```python
from build123d import *

# Parameters (mm, degrees)
BOSS_EXTRUDE1_DEPTH = 6.35
SKETCH2_R           = 1.5875
SKETCH2_W           = 80.264
SKETCH2_H           = 12.954
CUT_EXTRUDE1_DEPTH  = 224.053407282
SKETCH7_R           = 2.032
SKETCH7_R_2         = 1.651
SKETCH7_W           = 47.244
SKETCH7_H           = 139.192
CUT_EXTRUDE4_DEPTH  = 224.053407282
SKETCH8_R           = 1.651
CUT_EXTRUDE5_DEPTH  = 224.053407282
SKETCH9_R           = 1.778
CUT_EXTRUDE6_DEPTH  = 221.551312535


with BuildPart() as part:
    # Sketch1 → Boss-Extrude1 (new body)
    with BuildSketch(Plane(origin=(0, 0, 0), x_dir=(1, 0, 0), z_dir=(0, 1, 0))):
        with BuildLine():
            Line((-80, 112.5), (100, 112.5))
            Line((100, 112.5), (100, -112.5))
            Line((100, -112.5), (-80, -112.5))
            ThreePointArc((-80, -112.5), (-192.5, 0), (-80, 112.5))
        make_face()
    extrude(amount=-BOSS_EXTRUDE1_DEPTH)

    # Sketch2 → Cut-Extrude1 (cut, through all)
    with BuildSketch(Plane(origin=(0, 0, 0), x_dir=(1, 0, 0), z_dir=(0, 1, 0))):
        with Locations(Location((36.144045702, -66.3448, 0), (0, 0, 270))):
            Circle(SKETCH2_R)
        with Locations(Location((36.144045702, -59.9948, 0), (0, 0, 270))):
            Circle(SKETCH2_R)
        with Locations(Location((36.144045702, -53.6448, 0), (0, 0, 270))):
            Circle(SKETCH2_R)
        with Locations(Location((36.144045702, -47.2948, 0), (0, 0, 270))):
            Circle(SKETCH2_R)
        with Locations(Location((36.144045702, -40.9448, 0), (0, 0, 270))):
            Circle(SKETCH2_R)
        with Locations(Location((36.144045702, -34.5948, 0), (0, 0, 270))):
            Circle(SKETCH2_R)
        with Locations(Location((36.144045702, -28.2448, 0), (0, 0, 270))):
            Circle(SKETCH2_R)
        with Locations(Location((67.894045702, -66.3448, 0), (0, 0, 270))):
            Circle(SKETCH2_R)
        with Locations(Location((67.894045702, -59.9948, 0), (0, 0, 270))):
            Circle(SKETCH2_R)
        with Locations(Location((67.894045702, -53.6448, 0), (0, 0, 270))):
            Circle(SKETCH2_R)
        with Locations(Location((67.894045702, -47.2948, 0), (0, 0, 270))):
            Circle(SKETCH2_R)
        with Locations(Location((67.894045702, -40.9448, 0), (0, 0, 270))):
            Circle(SKETCH2_R)
        with Locations(Location((67.894045702, -34.5948, 0), (0, 0, 270))):
            Circle(SKETCH2_R)
        with Locations(Location((67.894045702, -28.2448, 0), (0, 0, 270))):
            Circle(SKETCH2_R)
        with Locations(Location((36.144045702, 66.3448, 0), (0, 0, 270))):
            Circle(SKETCH2_R)
        with Locations(Location((36.144045702, 59.9948, 0), (0, 0, 270))):
            Circle(SKETCH2_R)
        with Locations(Location((36.144045702, 53.6448, 0), (0, 0, 270))):
            Circle(SKETCH2_R)
        with Locations(Location((36.144045702, 47.2948, 0), (0, 0, 270))):
            Circle(SKETCH2_R)
        with Locations(Location((36.144045702, 40.9448, 0), (0, 0, 270))):
            Circle(SKETCH2_R)
        with Locations(Location((36.144045702, 34.5948, 0), (0, 0, 270))):
            Circle(SKETCH2_R)
        with Locations(Location((36.144045702, 28.2448, 0), (0, 0, 270))):
            Circle(SKETCH2_R)
        with Locations(Location((67.894045702, 66.3448, 0), (0, 0, 270))):
            Circle(SKETCH2_R)
        with Locations(Location((67.894045702, 59.9948, 0), (0, 0, 270))):
            Circle(SKETCH2_R)
        with Locations(Location((67.894045702, 53.6448, 0), (0, 0, 270))):
            Circle(SKETCH2_R)
        with Locations(Location((67.894045702, 47.2948, 0), (0, 0, 270))):
            Circle(SKETCH2_R)
        with Locations(Location((67.894045702, 40.9448, 0), (0, 0, 270))):
            Circle(SKETCH2_R)
        with Locations(Location((67.894045702, 34.5948, 0), (0, 0, 270))):
            Circle(SKETCH2_R)
        with Locations(Location((67.894045702, 28.2448, 0), (0, 0, 270))):
            Circle(SKETCH2_R)
        with Locations((52.019045702, -96.4438)):
            Rectangle(SKETCH2_W, SKETCH2_H)
        with Locations((52.019045702, 96.4438)):
            Rectangle(SKETCH2_W, SKETCH2_H)
    extrude(amount=-CUT_EXTRUDE1_DEPTH, mode=Mode.SUBTRACT)

    # Sketch7 → Cut-Extrude4 (cut, through all)
    with BuildSketch(Plane(origin=(0, 0, 0), x_dir=(1, 0, 0), z_dir=(0, 1, 0))):
        with Locations(Location((-50.421540267, 0, 0), (0, 0, 270))):
            Circle(SKETCH7_R)
        with Locations(Location((25.778459733, 0, 0), (0, 0, 270))):
            Circle(SKETCH7_R_2)
        with Locations(Location((86.738459733, 0, 0), (0, 0, 270))):
            Circle(SKETCH7_R_2)
        with Locations(Location((-50.421540267, 40.64, 0), (0, 0, 270))):
            Circle(SKETCH7_R_2)
        with Locations(Location((-50.421540267, -40.64, 0), (0, 0, 270))):
            Circle(SKETCH7_R_2)
        with Locations(Location((15.872459733, -40.64, 0), (0, 0, 270))):
            Circle(SKETCH7_R)
        with Locations(Location((15.872459733, 40.64, 0), (0, 0, 270))):
            Circle(SKETCH7_R)
        with Locations((-14.099540267, 0)):
            Rectangle(SKETCH7_W, SKETCH7_H)
    extrude(amount=-CUT_EXTRUDE4_DEPTH, mode=Mode.SUBTRACT)

    # Sketch8 → Cut-Extrude5 (cut, through all)
    with BuildSketch(Plane(origin=(0, 0, 0), x_dir=(1, 0, 0), z_dir=(0, 1, 0))):
        with Locations(Location((-177.3836, 33.02, 0), (0, 0, 270))):
            Circle(SKETCH8_R)
        with Locations(Location((-177.3836, -33.02, 0), (0, 0, 270))):
            Circle(SKETCH8_R)
        with Locations(Location((-151.9836, 33.02, 0), (0, 0, 270))):
            Circle(SKETCH8_R)
        with Locations(Location((-151.9836, -33.02, 0), (0, 0, 270))):
            Circle(SKETCH8_R)
        with BuildLine():
            Line((-167.0966, 25.4), (-229.776686608, 25.4))
            Line((-229.776686608, 25.4), (-229.776686608, -25.4))
            Line((-229.776686608, -25.4), (-167.0966, -25.4))
            ThreePointArc((-167.0966, -25.4), (-141.6966, 0), (-167.0966, 25.4))
        make_face()
    extrude(amount=-CUT_EXTRUDE5_DEPTH, mode=Mode.SUBTRACT)

    # Sketch9 → Cut-Extrude6 (cut, through all)
    with BuildSketch(Plane(origin=(0, 0, 0), x_dir=(1, 0, 0), z_dir=(0, 1, 0))):
        with Locations(Location((-161.795319669, -55.88, 0), (0, 0, 270))):
            Circle(SKETCH9_R)
        with Locations(Location((-124.964619687, -86.784626771, 0), (0, 0, 270))):
            Circle(SKETCH9_R)
        with Locations(Location((-161.795319669, 55.88, 0), (0, 0, 270))):
            Circle(SKETCH9_R)
        with Locations(Location((-124.964619687, 86.784626771, 0), (0, 0, 270))):
            Circle(SKETCH9_R)
    extrude(amount=-CUT_EXTRUDE6_DEPTH, mode=Mode.SUBTRACT)


solid = part.part
```
Geometry check sheet. Reference: the model listing, model coordinates, mm. A direction names the side the tool comes from. Coordinates: 2 decimals unless noted, no trailing zeros. Write each loop counter-clockwise with the first axis right and the second up, starting at its lowest first coordinate (ties: lowest second). Pieces come first, ordered by that corner, then holes. Notation, with made-up numbers: M -23,-36 L 19,-36 A23 cw 19,-24 Z; hole C 77.5,68.5 d2. An arc over 180 degrees is marked long. Use one line per item in the form item = value. Start each with the question number.
1) Section check D-D on y = -2. State how many separate pieces and enclosed holes the cut face has, and give its area (3 significant figures).
2) Release check for a two-part mould opening along X. For faces 4 (the flat face through (-14, -3, -69.596)), 5 (the flat face through (-43, -6.35, -2)), 6 (the cylindrical face through (-141.703, -3.131, 0.559)), 7 (the flat face through (100, -3, -2)) record: pulls with the +X half, pulls with the -X half, needs draft (parallel to the pull), parting line crosses it, or undercut.
3) Section check C-C on x = -16. Enter the section's corners in (y, z).
4) Thickness scan on probe 1 along Z at (x, y) = (20, -1); probe 2 along X at (y, z) = (-2, -35.5); probe 3 along Z at (x, y) = (-16, -1.75). Record the ranges inside material, lowest first. Write a range as from..to.
5) Section check A-A on x = 54. Enter the section's corners in (y, z), and give its area (3 significant figures).
6) Section check B-B on z = 93. Enter the section's corners in (x, y), and give its area (3 significant figures).
7) Set-up check for faces 1 (the flat face through (9, -3, -112.5)), 2 (the flat face through (-179, -3, 25.4)), 3 (the flat face through (9.522, -3, 1)): record each of +Z, -Z, +X, -X, +Y, -Y from which the full face is reachable in a straight line by a thin tool's end or side.
8) Go/stop test with flat-tipped pins: pin 1 Ø2 at (y, z) = (-3.5, 27) entering from -X; pin 2 Ø1 at (x, y) = (-81, -2.5) entering from +Z. Record where each tip stops, or that it passes through.
Responses:
q1.separate_pieces = 1
q1.enclosed_holes = 46
q1.area = 49,100 mm2
q2.face_4 = undercut
q2.face_5 = needs draft
q2.face_6 = pulls with the -X half
q2.face_7 = pulls with the +X half
q3.outline = M -6.35,-112.5 L 0,-112.5 L 0,-69.6 L -6.35,-69.6 Z; M -6.35,69.6 L 0,69.6 L 0,112.5 L -6.35,112.5 Z
q4.probe_1 = -112.5..-102.92, -89.97..89.97, 102.92..112.5
q4.probe_2 = -186.75..-37.72, 9.52..34.84, 37.45..66.59, 69.2..100
q4.probe_3 = -112.5..-69.6, 69.6..112.5
q5.outline = M -6.35,-112.5 L 0,-112.5 L 0,-102.92 L -6.35,-102.92 Z; M -6.35,-89.97 L 0,-89.97 L 0,89.97 L -6.35,89.97 Z; M -6.35,102.92 L 0,102.92 L 0,112.5 L -6.35,112.5 Z
q5.area = 1,260 mm2
q6.outline = M -143.3,-6.35 L 11.89,-6.35 L 11.89,0 L -143.3,0 Z; M 92.15,-6.35 L 100,-6.35 L 100,0 L 92.15,0 Z
q6.area = 1,040 mm2
q7.face_1 = -Z, +X, -X, +Y, -Y
q7.face_2 = -X, +Y, -Y
q7.face_3 = +Y, -Y
q8.pin_1 = -189.45
q8.pin_2 = 112.5
